Autodesk Inventor part; units mm, degrees
ref_plane "YZ Plane" through (0, 0, 0) normal (1, 0, 0) x (0, 1, 0)
ref_plane "XZ Plane" through (0, 0, 0) normal (0, 1, 0) x (-1, 0, 0)
ref_plane "XY Plane" through (0, 0, 0) normal (0, 0, 1) x (1, 0, 0)
sketch "Sketch1" plane through (0, 0, 0) normal (0, 1, 0) x (-1, 0, 0)
  line L0 (0, 0) -> (19.05, 0)
  line L1 (19.05, 0) -> (19.05, -50.8)
  line L2 (19.05, -50.8) -> (0, -50.8)
  line L3 (0, -50.8) -> (0, 0)
  dimension "d0" = 19.05
  dimension "d1" = 50.8
extrude "Extrusion1" add sketch "Sketch1" along normal blind 45.72
fillet "Fillet1" radius 25.4 1 edges at (-9.525, 0, -50.8)
sketch "Sketch2" plane through (0, 0, 0) normal (1, 0, 0) x (0, 0, -1)
  point P0 (0, 0)
sketch "Sketch4" plane through (-19.05, 0, 0) normal (0, 0, 1) x (1, 0, 0)
  line L0 (0, 0) -> (19.05, 0)
  line L1 (19.05, 0) -> (19.05, 6.3692)
  line L2 (19.05, 6.3692) -> (0, 6.3692)
  line L3 (0, 6.3692) -> (0, 0)
extrude "Extrusion3" add sketch "Sketch4" along normal blind 25.4
hole "Hole2" at (-9.525, 6.3692, 12.7) direction (0, -1, 0) diameter 9.525 end through all
hole "Hole3" at (0, 36.83, -25.4) direction (-1, 0, 0) diameter 9.525 end through all
pattern_linear "Rectangular Pattern1" count 2 spacing 25.4 along (0, -1, 0) of "Hole3"
properties part number "boxbeam gusset"
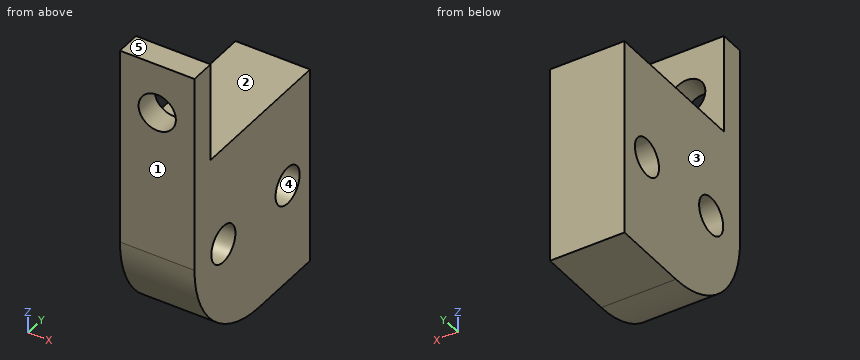
Could you check a few things on this model? Use its own coordinates, in mm. Face numbers are marked on the shaded views. A direction names the side the tool comes from. Coordinates: 2 decimals unless noted, no trailing zeros. Loops run counter-clockwise (first coordinate to the right, second up) from the corner with the lowest first, then second, coordinate; pieces in that order, holes last. Notation, with made-up numbers: (23, -39) -> (63, -39) arc R8 ccw to (63, -32) -> close; hole circle Ø8 at (5, -28). An arc over 180 degrees is marked (long way). Answer in a Markdown table with one row per item.
(1) Will these pins go through, and if not, where does the flat tip stop? pin 1 Ø1.5 at (x, y) = (-16.5, 15) entering from -Z; pin 2 Ø5.5 at (x, y) = (-9, 32.5) entering from +Z; pin 3 Ø1 at (x, z) = (-5.5, -37) entering from -Y.
Results found:
| item | result |
|---|---|
| pin 1 | stops at z = -48.9 |
| pin 2 | stops at z = 0 |
| pin 3 | stops at y = 2.55 |
(2) Imagine slicing it at A-A (y = 36.83). List the corners of the cut face in (x, z) for me, plus the area to 3 significant figures.
Results found:
| item | result |
|---|---|
| outline | (-19.05, -50.8) -> (0, -50.8) -> (0, -30.16) -> (-19.05, -30.16) -> close; (-19.05, -20.64) -> (0, -20.64) -> (0, 0) -> (-19.05, 0) -> close |
| area | 786 mm^2 |
(3) If I drill on probe 1 along Y at (x, z) = (-14, -25.4); probe 2 along Z at (x, y) = (-13.25, 36.83); probe 3 along Z at (x, y) = (-4.5, 11.43), over which ranges is the centre line in solid material (lowest first)?
Results found:
| item | result |
|---|---|
| probe 1 | y = 0 to 6.67, 16.19 to 32.07, 41.59 to 45.72 |
| probe 2 | z = -50.8 to -30.16, -20.64 to 0 |
| probe 3 | z = -46.61 to -30.16, -20.64 to 0 |
(4) Imagine slicing it at D-D (x = -1.5). List the corners of the cut face in (y, z) for me (1 decimal).
Results found:
| item | result |
|---|---|
| outline | (0, -25.4) arc R25.4 ccw to (25.4, -50.8) -> (45.7, -50.8) -> (45.7, 0) -> (6.4, 0) -> (6.4, 25.4) -> (0, 25.4) -> close; hole circle Ø9.5 at (11.4, -25.4); hole circle Ø9.5 at (36.8, -25.4) |
(5) Imagine slicing it at B-B (x = -8.75). List the corners of the cut face in (y, z) for me (1 decimal), plus the area to 3 significant figures.
Results found:
| item | result |
|---|---|
| outline | (0, -25.4) arc R25.4 ccw to (25.4, -50.8) -> (45.7, -50.8) -> (45.7, 0) -> (6.4, 0) -> (6.4, 8) -> (0, 8) -> close; (0, 17.4) -> (6.4, 17.4) -> (6.4, 25.4) -> (0, 25.4) -> close; hole circle Ø9.5 at (11.4, -25.4); hole circle Ø9.5 at (36.8, -25.4) |
| area | 2,140 mm^2 |
(6) Imagine slicing it at C-C (z = 12.7). List the corners of the cut face in (x, y) for me.
Results found:
| item | result |
|---|---|
| outline | (-19.05, 0) -> (-14.29, 0) -> (-14.29, 6.37) -> (-19.05, 6.37) -> close; (-4.76, 0) -> (0, 0) -> (0, 6.37) -> (-4.76, 6.37) -> close |
(7) For the marked faces 1 and 2, which set-ups out of +Z, -Z, +X, -X, +Y, -Y let a thin tool reach every point of the face, with its end or its side?
Results found:
| item | result |
|---|---|
| face 1 | +Z, -Z, +X, -X, -Y |
| face 2 | +Z, +X, -X, +Y |
(8) Thinking about a two-plate mould opening in Z: for the marked faces 3, 4 and 5, which applies, released by +Z, released by -Z, zero draft, split by the parting line, or undercut?
Results found:
| item | result |
|---|---|
| face 3 | zero draft |
| face 4 | undercut |
| face 5 | released by +Z |
